Part model, mm, in its own coordinate system. Face numbers are marked on the shaded views. A direction names the side the tool comes from. Coordinates: 2 decimals unless noted, no trailing zeros. Write each loop counter-clockwise with the first axis right and the second up, starting at its lowest first coordinate (ties: lowest second). Pieces come first, ordered by that corner, then holes. Notation, with made-up numbers: (36.5, -17.5) -> (52.5, -17.5) arc R21 cw to (52.5, 21.5) -> close; hole circle Ø3 at (79, 20.5). An arc over 180 degrees is marked (long way). One line per question, with ' | ' between items. Start each with the question number.
Item 1: Saw through at B-B (z = 1.5). List the corners of the cut face in (x, y), and give its area (3 significant figures).
Item 2: Pin check, flat tips, straight feed: pin 1 (6 mm diameter, centred on x = 1.5, z = 6, fed in from +Y); pin 2 (4 mm diameter, centred on x = -2, y = 0, fed in from -Z); pin 3 (0.8 mm diameter, centred on y = -5, z = 7, fed in from -X); pin 4 (1.9 mm diameter, centred on y = 7.5, z = 3, fed in from +X). Stop position of each tip, or through.
Item 3: Probe probe 1 along X at (y, z) = (4, 9.25); probe 2 along X at (y, z) = (0, -1); probe 3 along Y at (x, z) = (0, 2.25). List the from-to ranges inside material, lowest first. Write a range as [from, to].
Item 4: Saw through at A-A (y = -4.5). List the corners of the cut face in (x, z).
Item 5: Two-plate mould, pull along Y, no slides. Class the marked faces 1, 2 and 3: pulls with the +Y half, pulls with the -Y half, needs draft (parallel to the pull), parting line crosses it, or undercut.
Item 6: 3-axis set-ups, long thin cutter, end or side, ignore diameter. For the marked faces 4, 5 and 6: which of +Z, -Z, +X, -X, +Y, -Y reach the whole face in a straight line?
Item 7: Saw through at D-D (x = 0). List the corners of the cut face in (y, z).
Item 8: Saw through at C-C (y = -1.25). List the corners of the cut face in (x, z), and give its area (3 significant figures).
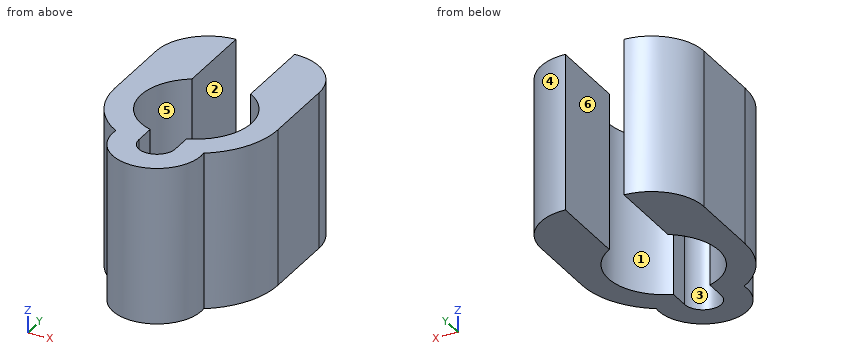
from build123d import *

# Parameters (mm, degrees)
BOSS_EXTRUDE1_DEPTH = 10
BOSS_EXTRUDE2_DEPTH = 2


with BuildPart() as part:
    # Sketch1 → Boss-Extrude1 (new body)
    with BuildSketch(Plane.XY):
        with BuildLine():
            Line((2.25, 5.018714975), (2.25, 3.605551275))
            ThreePointArc((2.25, 3.605551275), (4.223791394, -0.47126029), (1.4, -4.012792045))
            Line((1.4, -4.012792045), (1.4, -5.65))
            ThreePointArc((1.4, -5.65), (0, -7.05), (-1.4, -5.65))
            Line((-1.4, -5.65), (-1.4, -4.012792045))
            ThreePointArc((-1.4, -4.012792045), (-4.223791394, -0.47126029), (-2.25, 3.605551275))
            Line((-2.25, 3.605551275), (-2.25, 5.018714975))
            Line((-2.25, 5.018714975), (-2.25, 9.937240371))
            ThreePointArc((-2.25, 9.937240371), (-5.078427125, 8.765667496), (-6.25, 5.937240371))
            Line((-6.25, 5.937240371), (-6.25, 0))
            ThreePointArc((-6.25, 0), (-5.485043656, -2.996130185), (-3.377425252, -5.258849558))
            ThreePointArc((-3.377425252, -5.258849558), (0, -9.05), (3.377425252, -5.258849558))
            ThreePointArc((3.377425252, -5.258849558), (5.485043656, -2.996130185), (6.25, 0))
            Line((6.25, 0), (6.25, 5.937240371))
            ThreePointArc((6.25, 5.937240371), (5.078427125, 8.765667496), (2.25, 9.937240371))
            Line((2.25, 9.937240371), (2.25, 5.018714975))
        make_face()
    extrude(amount=BOSS_EXTRUDE1_DEPTH)

    # Sketch1_5 → Boss-Extrude2 (add)
    with BuildSketch(Plane.XY):
        with BuildLine():
            Line((2.25, 5.018714975), (2.25, 3.605551275))
            ThreePointArc((2.25, 3.605551275), (4.223791394, -0.47126029), (1.4, -4.012792045))
            Line((1.4, -4.012792045), (1.4, -5.65))
            ThreePointArc((1.4, -5.65), (0, -7.05), (-1.4, -5.65))
            Line((-1.4, -5.65), (-1.4, -4.012792045))
            ThreePointArc((-1.4, -4.012792045), (-4.223791394, -0.47126029), (-2.25, 3.605551275))
            Line((-2.25, 3.605551275), (-2.25, 5.018714975))
            Line((-2.25, 5.018714975), (-2.25, 9.937240371))
            ThreePointArc((-2.25, 9.937240371), (-5.078427125, 8.765667496), (-6.25, 5.937240371))
            Line((-6.25, 5.937240371), (-6.25, 0))
            ThreePointArc((-6.25, 0), (-5.485043656, -2.996130185), (-3.377425252, -5.258849558))
            ThreePointArc((-3.377425252, -5.258849558), (0, -9.05), (3.377425252, -5.258849558))
            ThreePointArc((3.377425252, -5.258849558), (5.485043656, -2.996130185), (6.25, 0))
            Line((6.25, 0), (6.25, 5.937240371))
            ThreePointArc((6.25, 5.937240371), (5.078427125, 8.765667496), (2.25, 9.937240371))
            Line((2.25, 9.937240371), (2.25, 5.018714975))
        make_face()
    extrude(amount=-BOSS_EXTRUDE2_DEPTH)


solid = part.part
From the geometry:
1) outline: (-6.25, 0) arc R6.25 ccw to (-3.38, -5.26) arc R3.4 ccw (long way) to (3.38, -5.26) arc R6.25 ccw to (6.25, 0) -> (6.25, 5.94) arc R4 ccw to (2.25, 9.94) -> (2.25, 3.61) arc R4.25 cw to (1.4, -4.01) -> (1.4, -5.65) arc R1.4 cw to (-1.4, -5.65) -> (-1.4, -4.01) arc R4.25 cw to (-2.25, 3.61) -> (-2.25, 9.94) arc R4 ccw to (-6.25, 5.94) -> close | area: 104 mm2
2) pin 1: y = 9.94 | pin 2: through | pin 3: x = -4.23 | pin 4: x = 6.2
3) probe 1: [-6.25, -2.25], [2.25, 6.25] | probe 2: [-6.25, -4.25], [4.25, 6.25] | probe 3: [-9.05, -7.05]
4) outline: (-4.34, -2) -> (-1.4, -2) -> (-1.4, 10) -> (-4.34, 10) -> close; (1.4, -2) -> (4.34, -2) -> (4.34, 10) -> (1.4, 10) -> close
5) face 1: undercut | face 2: needs draft | face 3: pulls with the +Y half
6) face 4: +Z, -Z, +X, +Y | face 5: +Z, -Z | face 6: +Z, -Z, +Y
7) outline: (-9.05, -2) -> (-7.05, -2) -> (-7.05, 10) -> (-9.05, 10) -> close
8) outline: (-6.12, -2) -> (-4.06, -2) -> (-4.06, 10) -> (-6.12, 10) -> close; (4.06, -2) -> (6.12, -2) -> (6.12, 10) -> (4.06, 10) -> close | area: 49.5 mm2
